from build123d import *

# Parameters (mm, degrees)
SKETCH1_R           = 18
BASEKEY_DEPTH       = 50
RECTANGLE_DEPTH     = 50
RECTANGLEPAT_COUNT  = 8
SKETCH_1_R          = 10
CUT_EXTRUDE_1_DEPTH = 22
CUT_EXTRUDE_2_DEPTH = 14


with BuildPart() as part:
    # Sketch1 → BaseKey (new, symmetric)
    with BuildSketch(Plane.XY):
        Circle(SKETCH1_R)
    extrude(amount=BASEKEY_DEPTH, both=True)

    # Sketch2 → Rectangle (add, symmetric)
    with BuildSketch(Plane.XY):
        with BuildLine():
            Line((-3.5, 19.691368668), (-3.5, 0))
            Line((-3.5, 0), (3.5, 0))
            Line((3.5, 0), (3.5, 19.691368668))
            ThreePointArc((3.5, 19.691368668), (0, 20), (-3.5, 19.691368668))
        make_face()
    rectangle = extrude(amount=RECTANGLE_DEPTH, both=True)

    # RectanglePat: Rectangle ×8 about axis
    rectanglepat_axis = Axis((0, 0, 0), (0, 0, 1))
    for i in range(1, RECTANGLEPAT_COUNT):
        add(rectangle.rotate(rectanglepat_axis, i * 360 / RECTANGLEPAT_COUNT))

    # 草图1 → 切除-拉伸1 (cut)
    with BuildSketch(Plane.XY.offset(50)):
        Circle(SKETCH_1_R)
    extrude(amount=-CUT_EXTRUDE_1_DEPTH, mode=Mode.SUBTRACT)

    # 草图2 → 切除-拉伸2 (cut)
    with BuildSketch(Plane(origin=(0, 0, 0), x_dir=(1, 0, 0), z_dir=(0, 1, 0))):
        Polygon((0, -50), (5, -50), (5, -43), (5, -36), (5, -28), (-5, -28), (-5, -36), (-5, -43), (-5, -50), align=None)
    extrude(amount=-CUT_EXTRUDE_2_DEPTH, mode=Mode.SUBTRACT)


solid = part.part
Input: part model. Units: mm. Frame: model coordinates. A direction names the side the tool comes from. Coordinates: 2 decimals unless noted, no trailing zeros. Write each loop counter-clockwise with the first axis right and the second up, starting at its lowest first coordinate (ties: lowest second). Pieces come first, ordered by that corner, then holes. Notation, with made-up numbers: M 11.25,47.5 L 70.25,47.5 A13 cw 70.25,66.5 Z; hole C -38,50.25 d2. An arc over 180 degrees is marked long. Answer as a JSON object with one key per item and string values. Group by question number.
(1) Section B-B on y = 0. Output: boundary loops of the cut face in (x, z).
(2) Mould query, pull axis Y, two halves, no side actions, for faces 6 (the face through (16.611, -6.934, 0.7)), 7 (the face through (-6.84, 16.65, 0.7)), 8 (the face through (-3.5, -19, 1)). Classes: pulls with the +Y half, pulls with the -Y half, needs draft (parallel to the pull), parting line crosses it, or undercut.
(3) Set-up query: faces 1 (the face through (19, -3.5, 1)), 2 (the face through (-16.611, 6.934, 0.7)), 3 (the face through (3.5, 19, 1)), 4 (the face through (-5, -11, 39)), 5 (the face through (6.934, 16.611, 0.7)). Return all of +Z, -Z, +X, -X, +Y, -Y with unobstructed straight access to the full face (end or side cutting, diameter ignored); none if empty.
(4) Section A-A on x = 0. Output: boundary loops of the cut face in (y, z), plus the area to 3 significant figures.
(5) Ray query, line 1 along Y through (x, z) = (0, 35); line 2 along Y through (x, z) = (-15.5, 8); line 3 along Y through (x, z) = (10, 15). Return the intervals inside material, ascending. Write a range as [from, to].
(6) Contact query for flat-ended pins moving along their axis: P1, Ø4.5, axis at y = -12, z = 38.5, coming from the +X side; P2, Ø8, axis at y = 8.5, z = -27, coming from the -X side; P3, Ø1.6, axis at y = -18.5, z = 1.5, coming from the +X side. Output: stop coordinate, or through.
Result set:
{
 "1": {"outline": "M -20,-50 L 20,-50 L 20,50 L 10,50 L 10,28 L -10,28 L -10,50 L -20,50 Z"},
 "2": {"face 6": "undercut", "face 7": "pulls with the +Y half", "face 8": "needs draft"},
 "3": {"face 1": "+Z, -Z, +X, -Y", "face 2": "+Z, -Z, -X", "face 3": "+Z, -Z, +X, +Y", "face 4": "+Z", "face 5": "+Z, -Z, +Y"},
 "4": {"outline": "M -20,-50 L 20,-50 L 20,50 L 10,50 L 10,28 L -14,28 L -14,50 L -20,50 Z", "area": "3,470 mm2"},
 "5": {"line 1": "y = [-20, -14], [10, 20]", "line 2": "y = [-12.64, -10.55], [-9.15, 9.15], [10.55, 12.64]", "line 3": "y = [-14.97, 14.97]"},
 "6": {"P1": "stops at x = 16.4", "P2": "stops at x = -17.43", "P3": "stops at x = 3.5"}
}
